from build123d import *

# Parameters (mm, degrees)
SKETCH1_R           = 1.5
BOSS_EXTRUDE1_DEPTH = 18
SKETCH2_R           = 2.5
BOSS_EXTRUDE2_DEPTH = 4
FILLET2_R           = 1
CUT_EXTRUDE2_DEPTH  = 3


with BuildPart() as part:
    # Sketch1 → Boss-Extrude1 (new body)
    with BuildSketch(Plane(origin=(0, 0, 0), x_dir=(1, 0, 0), z_dir=(0, 1, 0))):
        with Locations(Location((0, 0, 0), (0, 0, 270))):
            Circle(SKETCH1_R)
    extrude(amount=BOSS_EXTRUDE1_DEPTH)

    # Sketch2 → Boss-Extrude2 (add)
    with BuildSketch(Plane(origin=(0, 18, 0), x_dir=(1, 0, 0), z_dir=(0, 1, 0))):
        with Locations(Location((0, 0, 0), (0, 0, 270))):
            Circle(SKETCH2_R)
    extrude(amount=BOSS_EXTRUDE2_DEPTH)

    # Fillet2
    fillet2_edges = [part.edges().sort_by_distance(p)[0] for p in [
        (0, 22, -2.5),
    ]]
    fillet(fillet2_edges, radius=FILLET2_R)

    # Sketch3 → Cut-Extrude2 (cut)
    with BuildSketch(Plane(origin=(0, 22, 0), x_dir=(1, 0, 0), z_dir=(0, 1, 0))):
        Polygon((1.732050808, 0), (0.866025404, 1.5), (-0.866025404, 1.5), (-1.732050808, 0), (-0.866025404, -1.5), (0.866025404, -1.5), align=None)
    extrude(amount=-CUT_EXTRUDE2_DEPTH, mode=Mode.SUBTRACT)


solid = part.part
Input: part model. Units: mm. Frame: model coordinates. A direction names the side the tool comes from. Coordinates: 2 decimals unless noted, no trailing zeros. Write each loop counter-clockwise with the first axis right and the second up, starting at its lowest first coordinate (ties: lowest second). Pieces come first, ordered by that corner, then holes. Notation, with made-up numbers: M 21,20.5 L 31,20.5 A21 ccw 31,29.5 Z; hole C 34.25,70 d11. An arc over 180 degrees is marked long. Answer as a JSON object with one key per item and string values. Group by question number.
(1) Section A-A on x = 0. Output: boundary loops of the cut face in (y, z), plus the area to 3 significant figures.
(2) Contact query for flat-ended pins moving along their axis: P1, Ø1, axis at x = 0, z = 0.5, coming from the +Y side; P2, Ø0.9, axis at x = 0.5, y = 21, coming from the +Z side; P3, Ø1, axis at x = 0.5, y = 8, coming from the +Z side; P4, Ø2, axis at y = 14.5, z = 1.5, coming from the -X side. Output: stop coordinate, or through.
(3) Ray query, line 1 along Y through (x, z) = (0.45, -0.7); line 2 along X through (y, z) = (19.5, 0.25); line 3 along X through (y, z) = (15.25, -0.05). Return the intervals inside material, ascending. Write a range as [from, to].
(4) Mould query, pull axis X, two halves, no side actions, for faces 1 (the face through (-2.44, 19.48, -0.54)), 2 (the face through (0, 0, 0)), 3 (the face through (-1.305, 20.522, 0.74)). Classes: pulls with the +X half, pulls with the -X half, needs draft (parallel to the pull), parting line crosses it, or undercut.
(5) Set-up query: faces 4 (the face through (-2, 18, 0)), 5 (the face through (0, 21, 1.5)). Return all of +Z, -Z, +X, -X, +Y, -Y with unobstructed straight access to the full face (end or side cutting, diameter ignored); none if empty.
(6) Section B-B on y = 14.25. Output: boundary loops of the cut face in (x, z).
Result set:
{
 "1": {"outline": "M 0,-1.5 L 18,-1.5 L 18,-2.5 L 21,-2.5 A1 ccw 22,-1.5 L 19,-1.5 L 19,1.5 L 22,1.5 A1 ccw 21,2.5 L 18,2.5 L 18,1.5 L 0,1.5 Z", "area": "64.6 mm2"},
 "2": {"P1": "stops at y = 19", "P2": "stops at z = 2.5", "P3": "stops at z = 1.5", "P4": "stops at x = -1.41"},
 "3": {"line 1": "y = [0, 19]", "line 2": "x = [-2.49, -1.59], [1.59, 2.49]", "line 3": "x = [-1.5, 1.5]"},
 "4": {"face 1": "parting line crosses it", "face 2": "needs draft", "face 3": "undercut"},
 "5": {"face 4": "-Y", "face 5": "+Y"},
 "6": {"outline": "C 0,0 d3"}
}
